Autodesk Inventor part; units mm, degrees
ref_plane "YZ Plane" through (0, 0, 0) normal (1, 0, 0) x (0, 1, 0)
ref_plane "XZ Plane" through (0, 0, 0) normal (0, 1, 0) x (-1, 0, 0)
ref_plane "XY Plane" through (0, 0, 0) normal (0, 0, 1) x (1, 0, 0)
sketch "Skizze1" plane through (0, 0, 0) normal (0, 0, 1) x (1, 0, 0)
  line L0 (140.5121, 9.5998) -> (90.5121, 9.5998)
  line L1 (90.5121, 9.5998) -> (90.5121, 21.5998)
  line L2 (90.5121, 21.5998) -> (140.5121, 21.5998)
  line L3 (140.5121, 21.5998) -> (140.5121, 9.5998)
  point P0 (0, 0)
  dimension "d0" = 50
  dimension "d1" = 12
extrude "Extrusion1" add sketch "Skizze1" along normal blind 30
sketch "Skizze2" plane through (0, 0, 30) normal (0, 0, 1) x (1, 0, 0)
  line L0 (140.5121, 9.5998) -> (140.5121, 21.5998)
  line L1 (140.5121, 14.5998) -> (133.5121, 14.5998)
  line L2 (133.5121, 14.5998) -> (97.5121, 14.5998)
  line L3 (97.5121, 14.5998) -> (90.5121, 14.5998)
  line L4 (90.5121, 21.5998) -> (90.5121, 9.5998)
  line L5 (140.5121, 21.5998) -> (90.5121, 21.5998)
  point P0 (0, 0)
  dimension "d4" = 7
  dimension "d12" = 7
hole "Bohrung1" at (133.5121, 14.5998, 30) at (97.5121, 14.5998, 30) direction (0, 0, -1) diameter 4.3 end through all countersink diameter 9.4 countersink angle 90
sketch "Skizze4" plane through (90.5121, 21.5998, 0) normal (0, 1, 0) x (1, 0, 0)
  line L0 (25, -23) -> (25, -30)
  line L1 (50, -30) -> (0, -30)
  point P0 (-90.5121, 0)
  dimension "d37" = 7
hole "Bohrung5" at (115.5121, 21.5998, 23) direction (0, -1, 0) diameter 4.3 end through all countersink diameter 9.4 countersink angle 90
fillet "Rundung3" radius 2 5 edges at (140.5121, 15.5998, 30) (140.5121, 21.5998, 15) (115.5121, 21.5998, 30) (90.5121, 21.5998, 15) (90.5121, 15.5998, 30)
properties part number "HebelhalterBlock" material "Aluminium 6061(1)"
CAD build for the part. Positions are in the model's coordinates, mm. Round coordinates to 2 decimals unless told otherwise and drop trailing zeros. Loops run counter-clockwise (first coordinate to the right, second up) from the corner with the lowest first, then second, coordinate; pieces in that order, holes last. Notation, with made-up numbers: M 80,19 L 92,19 A19 cw 92,53 Z; hole C 17.5,9.25 d7. An arc over 180 degrees is marked long. One line per question, with ' | ' between items. Start each with the question number.
Item 1: Two-plate mould, pull along Z, no slides. Class faces 1 (the cylindrical face through (135.61, 15.07, 13.53)), 2 (the cylindrical face through (117.42, 14.26, 23.99)), 3 (the flat face through (115, 16, 0)): pulls with the +Z half, pulls with the -Z half, needs draft (parallel to the pull), parting line crosses it, or undercut.
Item 2: Cut at B-B, the plane z = 3.75. Write the cut outline in (x, y), plus the area to 3 significant figures.
Item 3: Cut at A-A, the plane z = 23. Write the cut outline in (x, y), plus the area to 3 significant figures.
Item 4: Cut at C-C, the plane y = 14.5. State how many separate pieces and enclosed holes the cut face has, plus the area to 3 significant figures.
Item 5: Wall check: line 1 (X direction, y = 16.5, z = 4.5); line 2 (X direction, y = 16, z = 18.25); line 3 (Y direction, x = 96, z = 8.5). Give the ranges that are in metal, low to high.
Item 6: Pin check, flat tips, straight feed: pin 1 Ø5.5 at (x, y) = (133.51, 14.6) entering from +Z; pin 2 Ø3 at (x, y) = (125.5, 13) entering from -Z. Stop position of each tip, or through.
Responses:
1) face 1: needs draft | face 2: undercut | face 3: pulls with the -Z half
2) outline: M 90.51,9.6 L 140.51,9.6 L 140.51,19.6 A2 ccw 138.51,21.6 L 92.51,21.6 A2 ccw 90.51,19.6 Z; hole C 97.51,14.6 d4.3; hole C 133.51,14.6 d4.3 | area: 569 mm²
3) outline: M 90.51,9.6 L 113.36,9.6 L 113.36,19.05 L 110.81,21.6 L 92.51,21.6 A2 ccw 90.51,19.6 Z; M 117.66,9.6 L 140.51,9.6 L 140.51,19.6 A2 ccw 138.51,21.6 L 120.21,21.6 L 117.66,19.05 Z; hole C 97.51,14.6 d4.3; hole C 133.51,14.6 d4.3 | area: 511 mm²
4) separate pieces: 3 | enclosed holes: 1 | area: 1,210 mm²
5) line 1: x = 90.51 to 96.51, 98.52 to 132.51, 134.52 to 140.51 | line 2: x = 90.51 to 95.88, 99.14 to 131.88, 135.14 to 140.51 | line 3: y = 9.6 to 13.07, 16.13 to 21.6
6) pin 1: stops at z = 28.05 | pin 2: stops at z = 0
